Source: CAD feature listing. Evaluate the final solid. Frame: model axes, mm. Give positions to 0.01 mm unless a question says otherwise; leave off trailing zeros. Order: outer loops, then holes, each group sorted by start corner. A loop starts at its lowest first (then second) coordinate and runs counter-clockwise, first axis right, second up. Notation, with made-up numbers: (-5, -15.75) - (42, -15.75) arc R37 ccw to (42, 22.25) - close; hole circle Ø3 at (77, -10.75). An arc over 180 degrees is marked (long way). One line per item, written item: value. Start each with the question number.
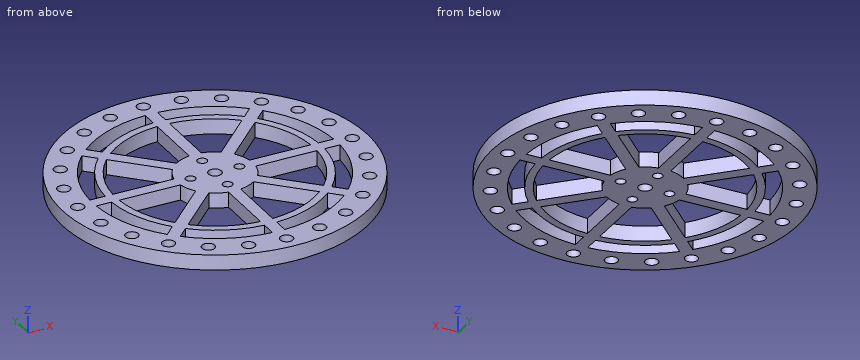
from build123d import *

# Parameters (mm, degrees)
SKETCH1_R           = 50
EXTRUDE2_DEPTH      = 2.5
EXTRUDE3_DEPTH      = 71.887234394
EXTRUDE3_DEPTH_BACK = 71.887234394
SKETCH2_R           = 2.1
EXTRUDE4_REACH      = 72.887
SKETCH3_R           = 1.6
SKETCH3_R_2         = 2.15


with BuildPart() as part:
    # Sketch1 → Extrude2 (new, symmetric)
    with BuildSketch(Plane.XY):
        Circle(SKETCH1_R)
        with BuildLine():
            Line((-2, 39.949968711), (-2, 34.942810419))
            ThreePointArc((-2, 34.942810419), (-13.393920133, 32.335783638), (-23.294084639, 26.122511764))
            Line((-23.294084639, 26.122511764), (-26.834680221, 29.663107346))
            ThreePointArc((-26.834680221, 29.663107346), (-15.307337295, 36.9551813), (-2, 39.949968711))
        make_face(mode=Mode.SUBTRACT)
        with BuildLine():
            Line((2, 34.942810419), (2, 39.949968711))
            ThreePointArc((2, 39.949968711), (15.307337295, 36.9551813), (26.834680221, 29.663107346))
            Line((26.834680221, 29.663107346), (23.294084639, 26.122511764))
            ThreePointArc((23.294084639, 26.122511764), (13.393920133, 32.335783638), (2, 34.942810419))
        make_face(mode=Mode.SUBTRACT)
        with BuildLine():
            Line((-29.663107346, 26.834680221), (-26.122511764, 23.294084639))
            ThreePointArc((-26.122511764, 23.294084639), (-32.335783638, 13.393920133), (-34.942810419, 2))
            Line((-34.942810419, 2), (-39.949968711, 2))
            ThreePointArc((-39.949968711, 2), (-36.9551813, 15.307337295), (-29.663107346, 26.834680221))
        make_face(mode=Mode.SUBTRACT)
        with BuildLine():
            Line((26.122511764, 23.294084639), (29.663107346, 26.834680221))
            ThreePointArc((29.663107346, 26.834680221), (36.9551813, 15.307337295), (39.949968711, 2))
            Line((39.949968711, 2), (34.942810419, 2))
            ThreePointArc((34.942810419, 2), (32.335783638, 13.393920133), (26.122511764, 23.294084639))
        make_face(mode=Mode.SUBTRACT)
        with BuildLine():
            Line((-39.949968711, -2), (-34.942810419, -2))
            ThreePointArc((-34.942810419, -2), (-32.335783638, -13.393920133), (-26.122511764, -23.294084639))
            Line((-26.122511764, -23.294084639), (-29.663107346, -26.834680221))
            ThreePointArc((-29.663107346, -26.834680221), (-36.9551813, -15.307337295), (-39.949968711, -2))
        make_face(mode=Mode.SUBTRACT)
        with BuildLine():
            Line((34.942810419, -2), (39.949968711, -2))
            ThreePointArc((39.949968711, -2), (36.9551813, -15.307337295), (29.663107346, -26.834680221))
            Line((29.663107346, -26.834680221), (26.122511764, -23.294084639))
            ThreePointArc((26.122511764, -23.294084639), (32.335783638, -13.393920133), (34.942810419, -2))
        make_face(mode=Mode.SUBTRACT)
        with BuildLine():
            Line((-26.834680221, -29.663107346), (-23.294084639, -26.122511764))
            ThreePointArc((-23.294084639, -26.122511764), (-13.393920133, -32.335783638), (-2, -34.942810419))
            Line((-2, -34.942810419), (-2, -39.949968711))
            ThreePointArc((-2, -39.949968711), (-15.307337295, -36.9551813), (-26.834680221, -29.663107346))
        make_face(mode=Mode.SUBTRACT)
        with BuildLine():
            Line((23.294084639, -26.122511764), (26.834680221, -29.663107346))
            ThreePointArc((26.834680221, -29.663107346), (15.307337295, -36.9551813), (2, -39.949968711))
            Line((2, -39.949968711), (2, -34.942810419))
            ThreePointArc((2, -34.942810419), (13.393920133, -32.335783638), (23.294084639, -26.122511764))
        make_face(mode=Mode.SUBTRACT)
        with BuildLine():
            ThreePointArc((-7.310750621, -10.139177746), (-4.783542905, -11.548494156), (-2, -12.338962679))
            Line((-2, -12.338962679), (-2, -32.438403167))
            ThreePointArc((-2, -32.438403167), (-12.437211552, -30.026084807), (-21.523201288, -24.351628412))
            Line((-21.523201288, -24.351628412), (-7.310750621, -10.139177746))
        make_face(mode=Mode.SUBTRACT)
        with BuildLine():
            ThreePointArc((-12.338962679, -2), (-11.548494156, -4.783542905), (-10.139177746, -7.310750621))
            Line((-10.139177746, -7.310750621), (-24.351628412, -21.523201288))
            ThreePointArc((-24.351628412, -21.523201288), (-30.026084807, -12.437211552), (-32.438403167, -2))
            Line((-32.438403167, -2), (-12.338962679, -2))
        make_face(mode=Mode.SUBTRACT)
        with BuildLine():
            ThreePointArc((21.523201288, -24.351628412), (12.437211552, -30.026084807), (2, -32.438403167))
            Line((2, -32.438403167), (2, -12.338962679))
            ThreePointArc((2, -12.338962679), (4.783542905, -11.548494156), (7.310750621, -10.139177746))
            Line((7.310750621, -10.139177746), (21.523201288, -24.351628412))
        make_face(mode=Mode.SUBTRACT)
        with BuildLine():
            ThreePointArc((32.438403167, -2), (30.026084807, -12.437211552), (24.351628412, -21.523201288))
            Line((24.351628412, -21.523201288), (10.139177746, -7.310750621))
            ThreePointArc((10.139177746, -7.310750621), (11.548494156, -4.783542905), (12.338962679, -2))
            Line((12.338962679, -2), (32.438403167, -2))
        make_face(mode=Mode.SUBTRACT)
        with BuildLine():
            ThreePointArc((-10.139177746, 7.310750621), (-11.548494156, 4.783542905), (-12.338962679, 2))
            Line((-12.338962679, 2), (-32.438403167, 2))
            ThreePointArc((-32.438403167, 2), (-30.026084807, 12.437211552), (-24.351628412, 21.523201288))
            Line((-24.351628412, 21.523201288), (-10.139177746, 7.310750621))
        make_face(mode=Mode.SUBTRACT)
        with BuildLine():
            ThreePointArc((-2, 12.338962679), (-4.783542905, 11.548494156), (-7.310750621, 10.139177746))
            Line((-7.310750621, 10.139177746), (-21.523201288, 24.351628412))
            ThreePointArc((-21.523201288, 24.351628412), (-12.437211552, 30.026084807), (-2, 32.438403167))
            Line((-2, 32.438403167), (-2, 12.338962679))
        make_face(mode=Mode.SUBTRACT)
        with BuildLine():
            ThreePointArc((24.351628412, 21.523201288), (30.026084807, 12.437211552), (32.438403167, 2))
            Line((32.438403167, 2), (12.338962679, 2))
            ThreePointArc((12.338962679, 2), (11.548494156, 4.783542905), (10.139177746, 7.310750621))
            Line((10.139177746, 7.310750621), (24.351628412, 21.523201288))
        make_face(mode=Mode.SUBTRACT)
        with BuildLine():
            ThreePointArc((2, 32.438403167), (12.437211552, 30.026084807), (21.523201288, 24.351628412))
            Line((21.523201288, 24.351628412), (7.310750621, 10.139177746))
            ThreePointArc((7.310750621, 10.139177746), (4.783542905, 11.548494156), (2, 12.338962679))
            Line((2, 12.338962679), (2, 32.438403167))
        make_face(mode=Mode.SUBTRACT)
    extrude(amount=EXTRUDE2_DEPTH, both=True)

    # Sketch2 → Extrude3 (cut, two sides: drawn at the far end of the back side and taken through both)
    with BuildSketch(Plane.XY.offset(2.5).offset(-EXTRUDE3_DEPTH_BACK)):
        with Locations((0, 45)):
            Circle(SKETCH2_R)
        with Locations((11.64685703, 43.466662183)):
            Circle(SKETCH2_R)
        with Locations((22.5, 38.97114317)):
            Circle(SKETCH2_R)
        with Locations((31.819805153, 31.819805153)):
            Circle(SKETCH2_R)
        with Locations((38.97114317, 22.5)):
            Circle(SKETCH2_R)
        with Locations((43.466662183, 11.64685703)):
            Circle(SKETCH2_R)
        with Locations((45, 0)):
            Circle(SKETCH2_R)
        with Locations((43.466662183, -11.64685703)):
            Circle(SKETCH2_R)
        with Locations((38.97114317, -22.5)):
            Circle(SKETCH2_R)
        with Locations((31.819805153, -31.819805153)):
            Circle(SKETCH2_R)
        with Locations((22.5, -38.97114317)):
            Circle(SKETCH2_R)
        with Locations((11.64685703, -43.466662183)):
            Circle(SKETCH2_R)
        with Locations((0, -45)):
            Circle(SKETCH2_R)
        with Locations((-11.64685703, -43.466662183)):
            Circle(SKETCH2_R)
        with Locations((-22.5, -38.97114317)):
            Circle(SKETCH2_R)
        with Locations((-31.819805153, -31.819805153)):
            Circle(SKETCH2_R)
        with Locations((-38.97114317, -22.5)):
            Circle(SKETCH2_R)
        with Locations((-43.466662183, -11.64685703)):
            Circle(SKETCH2_R)
        with Locations((-45, 0)):
            Circle(SKETCH2_R)
        with Locations((-43.466662183, 11.64685703)):
            Circle(SKETCH2_R)
        with Locations((-38.97114317, 22.5)):
            Circle(SKETCH2_R)
        with Locations((-31.819805153, 31.819805153)):
            Circle(SKETCH2_R)
        with Locations((-22.5, 38.97114317)):
            Circle(SKETCH2_R)
        with Locations((-11.64685703, 43.466662183)):
            Circle(SKETCH2_R)
    extrude(amount=EXTRUDE3_DEPTH + EXTRUDE3_DEPTH_BACK, mode=Mode.SUBTRACT)

    # Sketch3 → Extrude4 (cut, up to next)
    with BuildSketch(Plane.XY.offset(2.5), mode=Mode.PRIVATE) as extrude4_sk1:
        with Locations((0, 8)):
            Circle(SKETCH3_R)
    extrude4_tool1 = extrude(extrude4_sk1.sketch, amount=-EXTRUDE4_REACH, mode=Mode.PRIVATE) & part.part
    # Sketch3 → Extrude4 (cut, up to next)
    with BuildSketch(Plane.XY.offset(2.5), mode=Mode.PRIVATE) as extrude4_sk2:
        Circle(SKETCH3_R_2)
    extrude4_tool2 = extrude(extrude4_sk2.sketch, amount=-EXTRUDE4_REACH, mode=Mode.PRIVATE) & part.part
    # Sketch3 → Extrude4 (cut, up to next)
    with BuildSketch(Plane.XY.offset(2.5), mode=Mode.PRIVATE) as extrude4_sk3:
        with Locations((8, 0)):
            Circle(SKETCH3_R)
    extrude4_tool3 = extrude(extrude4_sk3.sketch, amount=-EXTRUDE4_REACH, mode=Mode.PRIVATE) & part.part
    # Sketch3 → Extrude4 (cut, up to next)
    with BuildSketch(Plane.XY.offset(2.5), mode=Mode.PRIVATE) as extrude4_sk4:
        with Locations((0, -8)):
            Circle(SKETCH3_R)
    extrude4_tool4 = extrude(extrude4_sk4.sketch, amount=-EXTRUDE4_REACH, mode=Mode.PRIVATE) & part.part
    # Sketch3 → Extrude4 (cut, up to next)
    with BuildSketch(Plane.XY.offset(2.5), mode=Mode.PRIVATE) as extrude4_sk5:
        with Locations((-8, 0)):
            Circle(SKETCH3_R)
    extrude4_tool5 = extrude(extrude4_sk5.sketch, amount=-EXTRUDE4_REACH, mode=Mode.PRIVATE) & part.part
    add(extrude4_tool1.solids().sort_by_distance((0, 8, 2.5))[0], mode=Mode.SUBTRACT)
    add(extrude4_tool2.solids().sort_by_distance((0, 0, 2.5))[0], mode=Mode.SUBTRACT)
    add(extrude4_tool3.solids().sort_by_distance((8, 0, 2.5))[0], mode=Mode.SUBTRACT)
    add(extrude4_tool4.solids().sort_by_distance((0, -8, 2.5))[0], mode=Mode.SUBTRACT)
    add(extrude4_tool5.solids().sort_by_distance((-8, 0, 2.5))[0], mode=Mode.SUBTRACT)


solid = part.part
1. Section B-B on y = 4.5. Return the cut outline in (x, z), then the cut area to 3 significant figures.
2. Section A-A on x = 0. Return the cut outline in (y, z).
3. Ray query, L1, parallel to Y at x = 0, z = 0.45; L2, parallel to X at y = -9, z = -1; L3, parallel to X at y = -5.5, z = 1.85. Return the intervals inside material, ascending.
4. Contact query for flat-ended pins moving along their axis: pin 1 Ø1.5 at (y, z) = (-26.5, 0) entering from +X; pin 2 Ø4 at (x, y) = (-22.5, -38.97) entering from -Z; pin 3 Ø2 at (x, z) = (-20.5, 1.5) entering from -Y; pin 4 Ø2.5 at (y, z) = (-19, 1) entering from -X. Output: stop coordinate, or through.
5. Section C-C on z = 1.15. Count the separate pieces of the cut face and the enclosed holes in it, then the cut area to 3 significant figures.
Data:
1. outline: (-49.8, -2.5) - (-39.75, -2.5) - (-39.75, 2.5) - (-49.8, 2.5) - close; (-34.71, -2.5) - (-32.19, -2.5) - (-32.19, 2.5) - (-34.71, 2.5) - close; (-11.66, -2.5) - (11.66, -2.5) - (11.66, 2.5) - (-11.66, 2.5) - close; (32.19, -2.5) - (34.71, -2.5) - (34.71, 2.5) - (32.19, 2.5) - close; (39.75, -2.5) - (49.8, -2.5) - (49.8, 2.5) - (39.75, 2.5) - close
1. area: 242 mm2
2. outline: (-50, -2.5) - (-47.1, -2.5) - (-47.1, 2.5) - (-50, 2.5) - close; (-42.9, -2.5) - (-9.6, -2.5) - (-9.6, 2.5) - (-42.9, 2.5) - close; (-6.4, -2.5) - (-2.15, -2.5) - (-2.15, 2.5) - (-6.4, 2.5) - close; (2.15, -2.5) - (6.4, -2.5) - (6.4, 2.5) - (2.15, 2.5) - close; (9.6, -2.5) - (42.9, -2.5) - (42.9, 2.5) - (9.6, 2.5) - close; (47.1, -2.5) - (50, -2.5) - (50, 2.5) - (47.1, 2.5) - close
3. L1: y = -50 to -47.1, -42.9 to -9.6, -6.4 to -2.15, 2.15 to 6.4, 9.6 to 42.9, 47.1 to 50
3. L2: x = -49.18 to -38.97, -33.82 to -31.23, -11.83 to -1.25, 1.25 to 11.83, 31.23 to 33.82, 38.97 to 49.18
3. L3: x = -49.7 to -39.62, -34.57 to -32.03, -11.22 to 11.22, 32.03 to 34.57, 39.62 to 49.7
4. pin 1: stops at x = 42.86
4. pin 2: passes through
4. pin 3: stops at y = -46.04
4. pin 4: stops at x = -46.74
5. separate pieces: 1
5. enclosed holes: 45
5. area: 4,270 mm2
